from build123d import *

# Parameters (mm, degrees)
F0_W     = 40
F0_H     = 8.5
F1_DEPTH = 8.5
F2_R     = 1.75
F3_DEPTH = 40
F2_R_2   = 3.5
F4_DEPTH = 4
F5_R     = 3.5
F6_DEPTH = 4
F7_R     = 0.6


with BuildPart() as f1:
    # F0 (on Top) → F1 (new body)
    with BuildSketch(Plane.XY):
        Rectangle(F0_W, F0_H)
    extrude(amount=F1_DEPTH)

    # F2 (on face) → F3 (cut)
    with BuildSketch(Plane.YZ.offset(20)):
        with Locations((0, 4.25)):
            Circle(F2_R)
    extrude(amount=-F3_DEPTH, mode=Mode.SUBTRACT)

    # F2 (on face) → F4 (cut)
    with BuildSketch(Plane.YZ.offset(20)):
        with Locations((0, 4.25)):
            Circle(F2_R_2)
        with Locations((0, 4.25)):
            Circle(F2_R, mode=Mode.SUBTRACT)
    extrude(amount=-F4_DEPTH, mode=Mode.SUBTRACT)

    # F5 (on face) → F6 (cut)
    with BuildSketch(Plane(origin=(-20, 0, 0), x_dir=(0, -1, 0), z_dir=(-1, 0, 0))):
        with Locations((0, 4.25)):
            Circle(F5_R)
    extrude(amount=-F6_DEPTH, mode=Mode.SUBTRACT)

    # F7
    f7_edges = [f1.edges().sort_by_distance(p)[0] for p in [
        (0, 4.25, 8.5),
        (0, 4.25, 0),
        (0, -4.25, 8.5),
        (0, -4.25, 0),
    ]]
    fillet(f7_edges, radius=F7_R)


solid = f1.part
Build history of the part. All positions in model axes, mm. A direction names the side the tool comes from. Round coordinates to 2 decimals unless told otherwise and drop trailing zeros. Write each loop counter-clockwise with the first axis right and the second up, starting at its lowest first coordinate (ties: lowest second). Pieces come first, ordered by that corner, then holes. Notation, with made-up numbers: (1, -13.75) -> (59, -13.75) arc R22 cw to (59, 18.25) -> close; hole circle Ø7 at (38, 40.5). An arc over 180 degrees is marked (long way). Write item = value, one per line.
(1) Tool access for faces 4 (the face through (-18.028, -1.615, 1.145)), 5 (the face through (0.22, -0.38, 2.54)), 6 (the face through (16, -2, 4)): list every direction of +Z, -Z, +X, -X, +Y, -Y with a clear straight run to the whole face (end or side of a thin tool).
Answer:
face_4 = -X
face_5 = +X, -X
face_6 = +X
(2) Band-saw the part on A-A (y = 0). Give the cut face in (x, z), then the cut area to 3 significant figures.
Answer:
outline = (-20, 0) -> (20, 0) -> (20, 0.75) -> (16, 0.75) -> (16, 2.5) -> (-16, 2.5) -> (-16, 0.75) -> (-20, 0.75) -> close; (-20, 7.75) -> (-16, 7.75) -> (-16, 6) -> (16, 6) -> (16, 7.75) -> (20, 7.75) -> (20, 8.5) -> (-20, 8.5) -> close
area = 172 mm2
(3) Band-saw the part on D-D (x = -9). Give the cut face in (y, z).
Answer:
outline = (-4.25, 0.6) arc R0.6 ccw to (-3.65, 0) -> (3.65, 0) arc R0.6 ccw to (4.25, 0.6) -> (4.25, 7.9) arc R0.6 ccw to (3.65, 8.5) -> (-3.65, 8.5) arc R0.6 ccw to (-4.25, 7.9) -> close; hole circle Ø3.5 at (0, 4.25)
(4) Band-saw the part on C-C (x = 17). Give the cut face in (y, z).
Answer:
outline = (-4.25, 0.6) arc R0.6 ccw to (-3.65, 0) -> (3.65, 0) arc R0.6 ccw to (4.25, 0.6) -> (4.25, 7.9) arc R0.6 ccw to (3.65, 8.5) -> (-3.65, 8.5) arc R0.6 ccw to (-4.25, 7.9) -> close; hole circle Ø7 at (0, 4.25)
(5) Probe L1, parallel to Z at x = 16.8, y = 0; L2, parallel to Z at x = -9, y = 0; L3, parallel to X at y = 3.25, z = 5. List the from-to ranges inside material, lowest first.
Answer:
L1 = 0 to 0.75, 7.75 to 8.5
L2 = 0 to 2.5, 6 to 8.5
L3 = -16 to 16
(6) Two-plate mould, pull along Y, no slides. Class faces 1 (the face through (-20, 4, 4)), 2 (the face through (0, -4.25, 4)), 3 (the face through (18.028, 1.615, 1.145)): pulls with the +Y half, pulls with the -Y half, needs draft (parallel to the pull), parting line crosses it, or undercut.
Answer:
face_1 = needs draft
face_2 = pulls with the -Y half
face_3 = undercut
(7) Flat gauge pins, fed straight in: pin 1 (4 mm diameter, centred on y = 0.5, z = 2.5, fed in from -X); pin 2 (4 mm diameter, centred on y = 0, z = 4.25, fed in from +X). Where does each tip first touch, or does it go through?
Answer:
pin_1 = -20
pin_2 = 16
(8) Band-saw the part on B-B (z = 4.25). Give the cut face in (x, y), then the cut area to 3 significant figures.
Answer:
outline = (-20, -4.25) -> (20, -4.25) -> (20, -3.5) -> (16, -3.5) -> (16, -1.75) -> (-16, -1.75) -> (-16, -3.5) -> (-20, -3.5) -> close; (-20, 3.5) -> (-16, 3.5) -> (-16, 1.75) -> (16, 1.75) -> (16, 3.5) -> (20, 3.5) -> (20, 4.25) -> (-20, 4.25) -> close
area = 172 mm2
